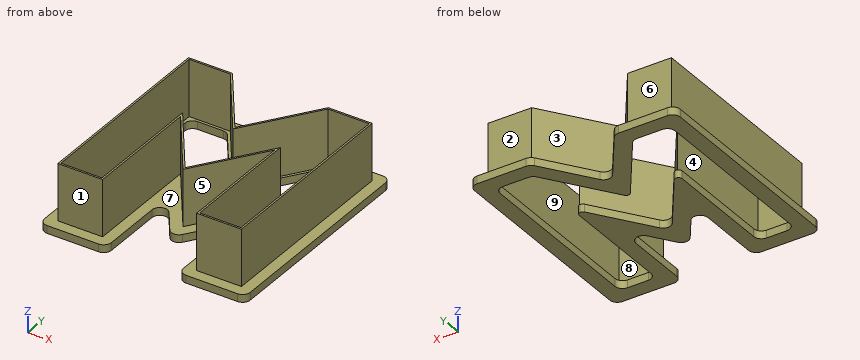
from build123d import *

# Parameters (mm, degrees)
F1_DEPTH = 3
F2_DEPTH = 25
F3_R     = 3
F4_R     = 1.4


with BuildPart() as f1:
    # F0 (on Top) → F1 (new body)
    with BuildSketch(Plane.XY):
        Polygon((-39.9790219963, 32.104852085), (-39.9790219963, -52.8951495448), (-13.9790203664, -52.8951495448), (-13.9790203664, -16.6482740563), (0, -36.6123841288), (13.9790203664, -16.6482740563), (13.9790203664, -52.8951495448), (39.9790219963, -52.8951495448), (39.9790219963, 32.104852085), (16.3761855044, 32.104852085), (0, 8.7172353989), (-16.3761855044, 32.104852085), align=None)
        Polygon((-18.2790211814, -48.5951487299), (-35.6790211814, -48.5951487299), (-35.6790211814, 27.8048512701), (-18.614624246, 27.8048512701), (0, 1.2204127569), (18.614624246, 27.8048512701), (35.6790211814, 27.8048512701), (35.6790211814, -48.5951487299), (18.2790211814, -48.5951487299), (18.2790211814, -3.0104138215), (0, -29.1155614869), (-18.2790211814, -3.0104138215), align=None, mode=Mode.SUBTRACT)
        Polygon((-35.6790211814, 27.8048512701), (-35.6790211814, -48.5951487299), (-18.2790211814, -48.5951487299), (-18.2790211814, -3.0104138215), (0, -29.1155614869), (18.2790211814, -3.0104138215), (18.2790211814, -48.5951487299), (35.6790211814, -48.5951487299), (35.6790211814, 27.8048512701), (18.614624246, 27.8048512701), (0, 1.2204127569), (-18.614624246, 27.8048512701), align=None)
        Polygon((-18.9790211814, -47.8951487299), (-34.9790211814, -47.8951487299), (-34.9790211814, 27.1048512701), (-18.9790211814, 27.1048512701), (0, 0), (18.9790211814, 27.1048512701), (34.9790211814, 27.1048512701), (34.9790211814, -47.8951487299), (18.9790211814, -47.8951487299), (18.9790211814, -0.7902974599), (0, -27.8951487299), (-18.9790211814, -0.7902974599), align=None, mode=Mode.SUBTRACT)
        Polygon((-34.9790211814, 27.1048512701), (-34.9790211814, -47.8951487299), (-18.9790211814, -47.8951487299), (-18.9790211814, -0.7902974599), (0, -27.8951487299), (18.9790211814, -0.7902974599), (18.9790211814, -47.8951487299), (34.9790211814, -47.8951487299), (34.9790211814, 27.1048512701), (18.9790211814, 27.1048512701), (0, 0), (-18.9790211814, 27.1048512701), align=None)
        Polygon((-19.9790211814, -46.8951487299), (-33.9790211814, -46.8951487299), (-33.9790211814, 26.1048512701), (-19.4995882319, 26.1048512701), (0, -1.7434467956), (19.4995882319, 26.1048512701), (33.9790211814, 26.1048512701), (33.9790211814, -46.8951487299), (19.9790211814, -46.8951487299), (19.9790211814, 2.3812973425), (0, -26.1517019343), (-19.9790211814, 2.3812973425), align=None, mode=Mode.SUBTRACT)
    extrude(amount=F1_DEPTH)

    # F0 (on Top) → F2 (join)
    with BuildSketch(Plane.XY):
        Polygon((-35.6790211814, 27.8048512701), (-35.6790211814, -48.5951487299), (-18.2790211814, -48.5951487299), (-18.2790211814, -3.0104138215), (0, -29.1155614869), (18.2790211814, -3.0104138215), (18.2790211814, -48.5951487299), (35.6790211814, -48.5951487299), (35.6790211814, 27.8048512701), (18.614624246, 27.8048512701), (0, 1.2204127569), (-18.614624246, 27.8048512701), align=None)
        Polygon((-18.9790211814, -47.8951487299), (-34.9790211814, -47.8951487299), (-34.9790211814, 27.1048512701), (-18.9790211814, 27.1048512701), (0, 0), (18.9790211814, 27.1048512701), (34.9790211814, 27.1048512701), (34.9790211814, -47.8951487299), (18.9790211814, -47.8951487299), (18.9790211814, -0.7902974599), (0, -27.8951487299), (-18.9790211814, -0.7902974599), align=None, mode=Mode.SUBTRACT)
    extrude(amount=F2_DEPTH)

    # F3
    f3_edges = [f1.edges().sort_by_distance(p)[0] for p in [
        (19.499588, 26.104851, 1.5),
        (33.979021, 26.104851, 1.5),
        (-33.979021, -46.895149, 1.5),
        (-19.979021, -46.895149, 1.5),
        (-39.979022, -52.89515, 1.5),
        (-13.97902, -52.89515, 1.5),
        (13.97902, -52.89515, 1.5),
        (39.979022, -52.89515, 1.5),
        (39.979022, 32.104852, 1.5),
        (16.376186, 32.104852, 1.5),
        (-16.376186, 32.104852, 1.5),
        (0, 8.717235, 1.5),
        (-39.979022, 32.104852, 1.5),
        (0, -36.612384, 1.5),
        (-13.97902, -16.648274, 1.5),
        (13.97902, -16.648274, 1.5),
        (0, -26.151702, 1.5),
        (-19.499588, 26.104851, 1.5),
        (-33.979021, 26.104851, 1.5),
        (33.979021, -46.895149, 1.5),
        (19.979021, -46.895149, 1.5),
    ]]
    fillet(f3_edges, radius=F3_R)

    # F4
    f4_edges = [f1.edges().sort_by_distance(p)[0] for p in [
        (-19.979021, 2.381297, 1.5),
        (19.979021, 2.381297, 1.5),
        (0, -1.743447, 1.5),
    ]]
    fillet(f4_edges, radius=F4_R)


solid = f1.part
Part model, mm, in its own coordinate system. Face numbers are marked on the shaded views. A direction names the side the tool comes from. Coordinates: 2 decimals unless noted, no trailing zeros. Order: outer loops, then holes, each group sorted by start corner. A loop starts at its lowest first (then second) coordinate and runs counter-clockwise, first axis right, second up. Notation, with made-up numbers: (58.5, 72) - (63.5, 72) arc R11 cw to (63.5, 88) - close; hole circle Ø10 at (48, 80). An arc over 180 degrees is marked (long way). Use CSV: the item, a comma, the result in double quotes.
Item 1: Probe probe 1 along X at (y, z) = (-35.5, 8); probe 2 along X at (y, z) = (6, 11.5); probe 3 along X at (y, z) = (-6, 22.75). List the from-to ranges inside material, lowest first.
Solved:
probe 1,"x = -35.68 to -34.98, -18.98 to -18.28, 18.28 to 18.98, 34.98 to 35.68"
probe 2,"x = -35.68 to -34.98, -4.2 to -3.35, 3.35 to 4.2, 34.98 to 35.68"
probe 3,"x = -35.68 to -34.98, -18.98 to -18.28, -16.19 to -15.33, 15.33 to 16.19, 18.28 to 18.98, 34.98 to 35.68"
Item 2: Saw through at B-B on z = 10.5. Give the cut face in (x, y).
Solved:
outline,"(-35.68, -48.6) - (-18.28, -48.6) - (-18.28, -3.01) - (0, -29.12) - (18.28, -3.01) - (18.28, -48.6) - (35.68, -48.6) - (35.68, 27.8) - (18.61, 27.8) - (0, 1.22) - (-18.61, 27.8) - (-35.68, 27.8) - close; hole (-34.98, -47.9) - (-18.98, -47.9) - (-18.98, -0.79) - (0, -27.9) - (18.98, -0.79) - (18.98, -47.9) - (34.98, -47.9) - (34.98, 27.1) - (18.98, 27.1) - (0, 0) - (-18.98, 27.1) - (-34.98, 27.1) - close"
Item 3: Saw through at D-D on y = -18. Give the number of separate pieces and of enclosed holes in the cut face, and give its area (3 significant figures).
Solved:
separate pieces,"4"
enclosed holes,"0"
area,"221 mm²"
Item 4: 3-axis set-ups, long thin cutter, end or side, ignore diameter. For the marked faces 1, 2, 3, 4 and 5: which of +Z, -Z, +X, -X, +Y, -Y reach the whole face in a straight line?
Solved:
face 1,"+Z, +X, -X, -Y"
face 2,"+Z, +X, -X, +Y"
face 3,"+Z, +Y"
face 4,"+Z"
face 5,"+Z, -Y"
Item 5: Mould opens along Y. For the marked faces 6, 7, 8 and 9 say: +Y half, -Y half, draft (parallel to the pull), parting line (faces both ways), or undercut.
Solved:
face 6,"+Y half"
face 7,"draft"
face 8,"undercut"
face 9,"undercut"
Item 6: Saw through at C-C on x = -5. Give the cut face in (y, z), and give its area (3 significant figures).
Solved:
outline,"(-29.47, 0) - (-19.01, 0) - (-19.01, 3) - (-20.75, 3) - (-20.75, 25) - (-21.97, 25) - (-21.97, 3) - (-29.47, 3) - close; (5.4, 0) - (15.86, 0) - (15.86, 3) - (8.36, 3) - (8.36, 25) - (7.14, 25) - (7.14, 3) - (5.4, 3) - close"
area,"116 mm²"
Item 7: Drop flat-ended pins along their axis: P1, Ø1.5, axis at y = -40.5, z = 19.5, coming from the -X side; P2, Ø1, axis at x = 16, z = 12, coming from the +Y side; P3, Ø5, axis at x = 23.5, z = 17, coming from the +Y side. Give the stop position or say it passes through.
Solved:
P1,"stops at x = -35.68"
P2,"stops at y = 24.78"
P3,"stops at y = 27.8"
Item 8: Saw through at A-A on x = -29.5. Give the cut face in (y, z), and give its area (3 significant figures).
Solved:
outline,"(-52.9, 0) - (-46.9, 0) - (-46.9, 3) - (-47.9, 3) - (-47.9, 25) - (-48.6, 25) - (-48.6, 3) - (-52.9, 3) - close; (26.1, 0) - (32.1, 0) - (32.1, 3) - (27.8, 3) - (27.8, 25) - (27.1, 25) - (27.1, 3) - (26.1, 3) - close"
area,"66.8 mm²"
